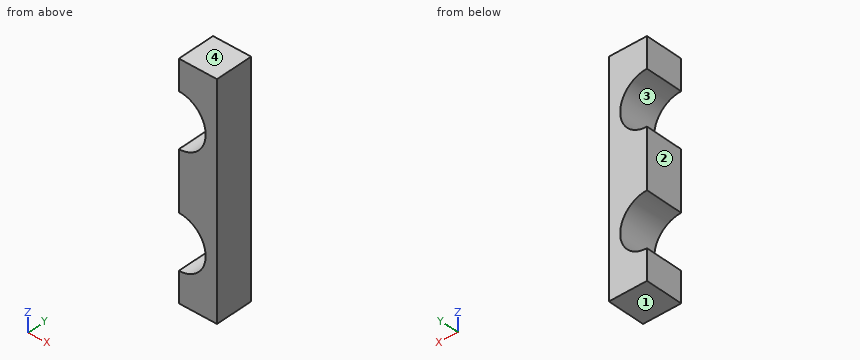
from build123d import *

# Parameters (mm, degrees)
EXTRUDE_1_DEPTH = 10


with BuildPart() as part:
    # Эскиз2 → Бобышка-Вытянуть1 (new body)
    with BuildSketch(Plane(origin=(0, 382.645061039, 0), x_dir=(1, 0, 0), z_dir=(0, 1, 0))):
        with BuildLine():
            Line((3.565848943, 102.773881836), (3.565848943, 110.773881836))
            Line((3.565848943, 110.773881836), (13.665848943, 110.773881836))
            Line((13.665848943, 110.773881836), (13.665848943, 50.773881836))
            Line((13.665848943, 50.773881836), (3.565848943, 50.773881836))
            Line((3.565848943, 50.773881836), (3.565848943, 58.773881836))
            ThreePointArc((3.565848943, 58.773881836), (10.665848943, 65.873881836), (3.565848943, 72.973881836))
            Line((3.565848943, 72.973881836), (3.565848943, 88.573881836))
            ThreePointArc((3.565848943, 88.573881836), (10.665848943, 95.673881836), (3.565848943, 102.773881836))
        make_face()
    extrude(amount=-EXTRUDE_1_DEPTH)


solid = part.part
Check sheet for the modelled part. Datum: model origin and axes. Units: mm. Face numbers are marked on the shaded views. Round coordinates to 2 decimals unless told otherwise and drop trailing zeros. Order: outer loops, then holes, each group sorted by start corner. A loop starts at its lowest first (then second) coordinate and runs counter-clockwise, first axis right, second up.
(1) Draft check along Z on the marked faces 1, 2, 3 and 4. Enter one of: pulls with the +Z half, pulls with the -Z half, needs draft (parallel to the pull), parting line crosses it, or undercut.
(2) Cross-section at B-B, the plane y = 377.75. Enter the section's corners in (x, z), and give its area (3 significant figures).
(3) Go/stop test with a flat-tipped pin: P1, Ø4, axis at y = 378, z = -68, coming from the -X side. Record where the tip stops, or that it passes through.
(4) Cross-section at A-A, the plane x = 5.5. Enter the section's corners in (y, z).
(5) Cross-section at D-D, the plane z = -63. Enter the section's corners in (x, y), and give its area (3 significant figures).
(6) Cross-section at C-C, the plane x = 10. Enter the section's corners in (y, z), and give its area (3 significant figures).
(7) Scan lines: probe 1 along Z at (x, y) = (5, 374.25); probe 2 along Z at (x, y) = (4.75, 377.75); probe 3 along X at (y, z) = (379.5, -99.5). Record each from-to range of solid material in increasing order.
Check sheet entries:
1. face 1: pulls with the -Z half
1. face 2: needs draft
1. face 3: undercut
1. face 4: pulls with the +Z half
2. outline: (3.57, -110.77) - (13.67, -110.77) - (13.67, -50.77) - (3.57, -50.77) - (3.57, -58.77) arc R7.1 cw to (3.57, -72.97) - (3.57, -88.57) arc R7.1 cw to (3.57, -102.77) - close
2. area: 448 mm2
3. P1: stops at x = 9.34
4. outline: (372.65, -110.77) - (382.65, -110.77) - (382.65, -102.51) - (372.65, -102.51) - close; (372.65, -88.84) - (382.65, -88.84) - (382.65, -72.71) - (372.65, -72.71) - close; (372.65, -59.04) - (382.65, -59.04) - (382.65, -50.77) - (372.65, -50.77) - close
5. outline: (10.06, 372.65) - (13.67, 372.65) - (13.67, 382.65) - (10.06, 382.65) - close
5. area: 36.1 mm2
6. outline: (372.65, -110.77) - (382.65, -110.77) - (382.65, -98.68) - (372.65, -98.68) - close; (372.65, -92.67) - (382.65, -92.67) - (382.65, -68.88) - (372.65, -68.88) - close; (372.65, -62.87) - (382.65, -62.87) - (382.65, -50.77) - (372.65, -50.77) - close
6. area: 480 mm2
7. probe 1: z = -110.77 to -102.63, -88.72 to -72.83, -58.92 to -50.77
7. probe 2: z = -110.77 to -102.67, -88.67 to -72.87, -58.87 to -50.77
7. probe 3: x = 9.55 to 13.67
